```python
from build123d import *

# Parameters (mm, degrees)
SKETCH1_W               = 38.1
SKETCH1_H               = 20.32
BOSS_EXTRUDE1_DEPTH     = 1.524
F_4_CLEARANCE_HOLE1_D   = 3.2639
SKETCH4_W               = 4.572
SKETCH4_H               = 6.096
BOSS_EXTRUDE2_DEPTH     = 4.064
SKETCH5_R               = 5.969
BOSS_EXTRUDE3_DEPTH     = 6.604
SKETCH6_W               = 10.668
SKETCH6_H               = 13.462
BOSS_EXTRUDE4_DEPTH     = 4.826
BOSS_EXTRUDE5_DEPTH     = 10.668
SKETCH8_W               = 7.874
SKETCH8_H               = 5.588
BOSS_EXTRUDE6_DEPTH     = 3.048
SKETCH9_W               = 7.112
SKETCH9_H               = 5.08
BOSS_EXTRUDE7_DEPTH     = 1.524
SKETCH10_W              = 2.54
SKETCH10_H              = 4.064
BOSS_EXTRUDE8_DEPTH     = 1.016
SKETCH11_W              = 5.08
SKETCH11_H              = 5.08
BOSS_EXTRUDE9_DEPTH     = 1.016
SKETCH12_W              = 4.064
SKETCH12_H              = 2.032
BOSS_EXTRUDE10_DEPTH    = 1.016
SKETCH13_W              = 3.048
SKETCH13_H              = 3.048
BOSS_EXTRUDE11_DEPTH    = 0.508
SKETCH14_W              = 3.048
SKETCH14_H              = 3.556
BOSS_EXTRUDE12_DEPTH    = 1.016
SKETCH15_W              = 2.032
SKETCH15_H              = 4.064
BOSS_EXTRUDE13_DEPTH    = 1.524
SKETCH16_W              = 3.048
SKETCH16_H              = 3.048
BOSS_EXTRUDE14_DEPTH    = 1.016
SKETCH17_R              = 0.508
BOSS_EXTRUDE15_DEPTH    = 1.524
LPATTERN1_COUNT         = 4
LPATTERN1_PITCH         = 2.794
MIRROR1_COPY_1_SKETCH_R = 0.508
MIRROR1_COPY_1_DEPTH    = 1.524
MIRROR1_COPY_2_SKETCH_R = 0.508
MIRROR1_COPY_2_DEPTH    = 1.524
MIRROR1_COPY_3_SKETCH_R = 0.508
MIRROR1_COPY_3_DEPTH    = 1.524
SKETCH22_W              = 13.60805
SKETCH22_H              = 0.79375
CUT_EXTRUDE2_DEPTH      = 1.524
SKETCH24_W              = 4.064
SKETCH24_H              = 5.588
CUT_EXTRUDE3_DEPTH      = 3.556
SKETCH25_W              = 0.381
SKETCH25_H              = 0.381
BOSS_EXTRUDE16_DEPTH    = 3.048
CHAMFER1_SIZE           = 0.127
CUT_EXTRUDE4_DEPTH      = 0.254
CHAMFER2_SIZE           = 1.778
CHAMFER2_SIZE2          = 2.737879906
CHAMFER2_PART_2_SIZE    = 1.778
CHAMFER2_PART_2_SIZE2   = 2.737879906


with BuildPart() as part:
    # Sketch1 → Boss-Extrude1 (new body)
    with BuildSketch(Plane(origin=(0, 0, 0), x_dir=(1, 0, 0), z_dir=(0, 1, 0))):
        Rectangle(SKETCH1_W, SKETCH1_H)
    extrude(amount=BOSS_EXTRUDE1_DEPTH)

    # #4 Clearance Hole1 (through all)
    with Locations(Plane(origin=(0, 1.524, 0), x_dir=(1, 0, 0), z_dir=(0, 1, 0))):
        with Locations((-15.875, 6.985), (15.875, -6.985), (-15.875, -6.985), (15.875, 6.985)):
            Hole(F_4_CLEARANCE_HOLE1_D / 2)

    # Sketch4 → Boss-Extrude2 (add)
    with BuildSketch(Plane(origin=(0, 1.524, 0), x_dir=(1, 0, 0), z_dir=(0, 1, 0))):
        with Locations((-16.764, 0)):
            Rectangle(SKETCH4_W, SKETCH4_H)
    extrude(amount=BOSS_EXTRUDE2_DEPTH)

    # Sketch5 → Boss-Extrude3 (add)
    with BuildSketch(Plane(origin=(0, 1.524, 0), x_dir=(1, 0, 0), z_dir=(0, 1, 0))):
        with Locations((8.89, 0)):
            Circle(SKETCH5_R)
    extrude(amount=BOSS_EXTRUDE3_DEPTH)

    # Sketch6 → Boss-Extrude4 (add)
    with BuildSketch(Plane(origin=(0, 1.524, 0), x_dir=(1, 0, 0), z_dir=(0, 1, 0))):
        with Locations((-7.239, 0)):
            Rectangle(SKETCH6_W, SKETCH6_H)
    extrude(amount=BOSS_EXTRUDE4_DEPTH)

    # Sketch7 → Boss-Extrude5 (add)
    with BuildSketch(Plane.ZY.offset(12.573)):
        Polygon((-6.731, 6.35), (-4.953, 9.906), (-1.651, 9.906), (-1.651, 6.35), align=None)
        Polygon((6.731, 6.35), (4.953, 9.906), (1.651, 9.906), (1.651, 6.35), align=None)
    extrude(amount=-BOSS_EXTRUDE5_DEPTH)

    # Sketch8 → Boss-Extrude6 (add)
    with BuildSketch(Plane.XZ):
        with Locations((7.239, -7.366)):
            Rectangle(SKETCH8_W, SKETCH8_H)
    extrude(amount=BOSS_EXTRUDE6_DEPTH)

    # Sketch9 → Boss-Extrude7 (add)
    with BuildSketch(Plane.XZ):
        with Locations((7.239, 7.62)):
            Rectangle(SKETCH9_W, SKETCH9_H)
    extrude(amount=BOSS_EXTRUDE7_DEPTH)

    # Sketch10 → Boss-Extrude8 (add)
    with BuildSketch(Plane.XZ):
        with Locations((13.589, 0)):
            Rectangle(SKETCH10_W, SKETCH10_H)
    extrude(amount=BOSS_EXTRUDE8_DEPTH)

    # Sketch11 → Boss-Extrude9 (add)
    with BuildSketch(Plane.XZ):
        with Locations((4.191, 0)):
            Rectangle(SKETCH11_W, SKETCH11_H)
    extrude(amount=BOSS_EXTRUDE9_DEPTH)

    # Sketch12 → Boss-Extrude10 (add)
    with BuildSketch(Plane.XZ):
        with Locations((-2.413, 7.112)):
            Rectangle(SKETCH12_W, SKETCH12_H)
    extrude(amount=BOSS_EXTRUDE10_DEPTH)

    # Sketch13 → Boss-Extrude11 (add)
    with BuildSketch(Plane.XZ):
        with Locations((-3.81, -6.096)):
            Rectangle(SKETCH13_W, SKETCH13_H)
    extrude(amount=BOSS_EXTRUDE11_DEPTH)

    # Sketch14 → Boss-Extrude12 (add)
    with BuildSketch(Plane.XZ):
        with Locations((-9.906, -6.35)):
            Rectangle(SKETCH14_W, SKETCH14_H)
    extrude(amount=BOSS_EXTRUDE12_DEPTH)

    # Sketch15 → Boss-Extrude13 (add)
    with BuildSketch(Plane.XZ):
        with Locations((-15.494, 1.27)):
            Rectangle(SKETCH15_W, SKETCH15_H)
    extrude(amount=BOSS_EXTRUDE13_DEPTH)

    # Sketch16 → Boss-Extrude14 (add)
    with BuildSketch(Plane.XZ):
        with Locations((-9.398, 0)):
            Rectangle(SKETCH16_W, SKETCH16_H)
    extrude(amount=BOSS_EXTRUDE14_DEPTH)

    # Sketch17 → Boss-Extrude15 (add)
    with BuildSketch(Plane.XZ):
        with Locations((-11.684, -3.556)):
            Circle(SKETCH17_R)
    boss_extrude15 = extrude(amount=BOSS_EXTRUDE15_DEPTH)

    # LPattern1: Boss-Extrude15 ×4
    with Locations(*[(i * LPATTERN1_PITCH, 0, 0) for i in range(1, LPATTERN1_COUNT)]):
        add(boss_extrude15)

    # Mirror1: Boss-Extrude15 across plane
    add(boss_extrude15.mirror(Plane.XY))

    # Mirror1 copy 1 sketch → Mirror1 copy 1 (add)
    with BuildSketch(Plane(origin=(2.794, 0, 0), x_dir=(1, 0, 0), z_dir=(0, -1, 0))):
        with Locations((-11.684, 3.556)):
            Circle(MIRROR1_COPY_1_SKETCH_R)
    extrude(amount=MIRROR1_COPY_1_DEPTH)

    # Mirror1 copy 2 sketch → Mirror1 copy 2 (add)
    with BuildSketch(Plane(origin=(5.588, 0, 0), x_dir=(1, 0, 0), z_dir=(0, -1, 0))):
        with Locations((-11.684, 3.556)):
            Circle(MIRROR1_COPY_2_SKETCH_R)
    extrude(amount=MIRROR1_COPY_2_DEPTH)

    # Mirror1 copy 3 sketch → Mirror1 copy 3 (add)
    with BuildSketch(Plane(origin=(8.382, 0, 0), x_dir=(1, 0, 0), z_dir=(0, -1, 0))):
        with Locations((-11.684, 3.556)):
            Circle(MIRROR1_COPY_3_SKETCH_R)
    extrude(amount=MIRROR1_COPY_3_DEPTH)

    # Sketch22 → Cut-Extrude2 (cut)
    with BuildSketch(Plane(origin=(0, 1.524, 0), x_dir=(1, 0, 0), z_dir=(0, 1, 0))):
        with Locations((7.439025, 9.763125)):
            Rectangle(SKETCH22_W, SKETCH22_H)
    extrude(amount=-CUT_EXTRUDE2_DEPTH, mode=Mode.SUBTRACT)

    # Sketch24 → Cut-Extrude3 (cut)
    with BuildSketch(Plane(origin=(0, 5.588, 0), x_dir=(1, 0, 0), z_dir=(0, 1, 0))):
        with Locations((-16.764, 0)):
            Rectangle(SKETCH24_W, SKETCH24_H)
    extrude(amount=-CUT_EXTRUDE3_DEPTH, mode=Mode.SUBTRACT)

    # Sketch25 → Boss-Extrude16 (add)
    with BuildSketch(Plane(origin=(0, 2.032, 0), x_dir=(1, 0, 0), z_dir=(0, 1, 0))):
        with Locations((-17.018, 1.3335)):
            Rectangle(SKETCH25_W, SKETCH25_H)
        with Locations((-17.018, -1.3335)):
            Rectangle(SKETCH25_W, SKETCH25_H)
    extrude(amount=BOSS_EXTRUDE16_DEPTH)

    # Chamfer1
    chamfer1_edges = [part.edges().sort_by_distance(p)[0] for p in [
        (-17.018, 5.08, -1.524),
        (-17.2085, 5.08, -1.3335),
        (-17.018, 5.08, -1.143),
        (-16.8275, 5.08, -1.3335),
        (-17.018, 5.08, 1.143),
        (-17.2085, 5.08, 1.3335),
        (-17.018, 5.08, 1.524),
        (-16.8275, 5.08, 1.3335),
    ]]
    chamfer(chamfer1_edges, length=CHAMFER1_SIZE)

    # Sketch26 → Cut-Extrude4 (cut)
    with BuildSketch(Plane.ZY.offset(19.05)):
        Polygon((-0.9525, 5.588), (-0.381, 5.0165), (-0.381, 2.286), (0.381, 2.286), (0.381, 5.0165), (0.9525, 5.588), align=None)
    extrude(amount=-CUT_EXTRUDE4_DEPTH, mode=Mode.SUBTRACT)

    # Chamfer2
    chamfer2_edges = [part.edges().sort_by_distance(p)[0] for p in [
        (3.302, -3.048, -7.366),
    ]]
    chamfer2_side = [part.faces().sort_by_distance(p)[0] for p in [
        (3.302, -1.524, -7.366),
    ]]
    chamfer(chamfer2_edges, length=CHAMFER2_SIZE, length2=CHAMFER2_SIZE2, reference=chamfer2_side[0])

    # Chamfer2 part 2
    chamfer2_part_2_edges = [part.edges().sort_by_distance(p)[0] for p in [
        (11.176, -3.048, -7.366),
    ]]
    chamfer2_part_2_side = [part.faces().sort_by_distance(p)[0] for p in [
        (11.176, -1.524, -7.366),
    ]]
    chamfer(chamfer2_part_2_edges, length=CHAMFER2_PART_2_SIZE, length2=CHAMFER2_PART_2_SIZE2, reference=chamfer2_part_2_side[0])


solid = part.part
```
Read the model definition and answer for the solid it produces. Units are mm, in the model's axes. A direction names the side the tool comes from. Give positions to 0.01 mm unless a question says otherwise; leave off trailing zeros. Order: outer loops, then holes, each group sorted by start corner. A loop starts at its lowest first (then second) coordinate and runs counter-clockwise, first axis right, second up. Notation, with made-up numbers: (-25, -39) -> (1, -39) arc R23 cw to (1, -15) -> close; hole circle Ø8 at (-5, 35.5). An arc over 180 degrees is marked (long way). One line per item, written item: value. Start each with the question number.
(1) The part is cut by section D-D (z = 7.75). Determine the outline of the cut face in (x, y) (3 decimals), and give its area (3 significant figures).
(2) The part is cut by section C-C (x = 15.5). Determine the outline of the cut face in (y, z), and give its area (3 significant figures).
(3) A tool of negligible diameter and unlimited length cuts with its end or side. For faces 4 (the flat face through (12.319, -0.5, 0)), 5 (the flat face through (-14.732, 4, 0)), 6 (the flat face through (-3.3, -1.524, 3.6)), 7 (the flat face through (7, -1, -10.16)), 8 (the cylindrical face through (-11.215, -0.751, -3.751)), from which of +Z, -Z, +X, -X, +Y, -Y can it reach the whole face along a straight path? Write none if from no direction.
(4) The part is cut by section A-A (y = 3.5). State how many separate pieces and enclosed holes the cut face has, and give its area (3 significant figures).
(5) For a pull along X with two mould halves and no side action, classify faces 1 (the cylindrical face through (-5.627, -0.751, -3.751)), 2 (the flat face through (19.05, 1, 0)), 3 (the flat face through (-7, 8, -1.651)) as released by +X, released by -X, zero draft, split by the parting line, or undercut.
(6) Straight lines are drawn through the part: L1, parallel to X at y = 5, z = -0.25 (3 decimals); L2, parallel to X at y = 3.5, z = -2.5 (3 decimals); L3, parallel to Y at x = -10, z = 4. For each, find the intervals that lie inside material, in ascending order.
(7) Flat-ended cylindrical pins translate along their axes: P1, Ø1.1, axis at x = -6, z = -3.5, coming from the -Y side; P2, Ø3, axis at x = -6, y = 8.5, coming from the +Z side; P3, Ø3, axis at x = -17, y = 3.5, coming from the -Z side; P4, Ø2.5, axis at x = -5.5, z = -0.5, coming from the +Y side. Find the tip coordinate at first contact, or state that the pin passes through.
Taken from the geometry:
1. outline: (-19.05, 0) -> (-17.317, 0) -> (-17.317, 1.524) -> (-19.05, 1.524) -> close; (-14.433, 0) -> (-4.445, 0) -> (-4.445, -1.016) -> (-0.381, -1.016) -> (-0.381, 0) -> (3.683, 0) -> (3.683, -1.524) -> (10.795, -1.524) -> (10.795, 0) -> (14.433, 0) -> (14.433, 1.524) -> (-14.433, 1.524) -> close; (17.317, 0) -> (19.05, 0) -> (19.05, 1.524) -> (17.317, 1.524) -> close
1. area: 64.2 mm^2
2. outline: (0, -10.16) -> (1.52, -10.16) -> (1.52, -8.57) -> (0, -8.57) -> close; (0, -5.4) -> (1.52, -5.4) -> (1.52, 5.4) -> (0, 5.4) -> close; (0, 8.57) -> (1.52, 8.57) -> (1.52, 10.16) -> (0, 10.16) -> close
2. area: 21.3 mm^2
3. face 4: +Z, -Z, -Y
3. face 5: +Y
3. face 6: +Z, -Z, +X, -X, -Y
3. face 7: -Z, +X, -X, +Y, -Y
3. face 8: -Y
4. separate pieces: 5
4. enclosed holes: 0
4. area: 261 mm^2
5. face 1: undercut
5. face 2: released by +X
5. face 3: zero draft
6. L1: -14.732 to -14.478, -12.573 to -1.905, 2.926 to 14.854
6. L2: -19.05 to -18.796, -14.732 to -14.478, -12.573 to -1.905, 3.47 to 14.31
6. L3: 0 to 9.91
7. P1: y = -1.52
7. P2: z = 6.41
7. P3: z = -3.05
7. P4: y = 9.91
